For this review, use the dimensioned drawing (mm, ordinates from the lowest corner) and the shaded views. A direction names the side the tool comes from. Round coordinates to 2 decimals unless told otherwise and drop trailing zeros. Loops run counter-clockwise (first coordinate to the right, second up) from the corner with the lowest first, then second, coordinate; pieces in that order, holes last. Notation, with made-up numbers: (10, 45.5) - (34, 45.5) arc R29 ccw to (34, 70.5) - close; hole circle Ø10 at (80.5, 73.25). An arc over 180 degrees is marked (long way). Answer as CSV lines item,"result". Start each with the question number.
(1) For the marked faces 4, 5 and 6, list the 3-axis set-ups (+Z, -Z, +X, -X, +Y, -Y) from which the entire face can be reached by the end or side of a thin tool; tool diameter is ignored.
(2) For P1, Ø2, axis at y = 47.5, z = 2, coming from the +X side; P2, Ø1, axis at y = 53.5, z = 2, coming from the -X side, all flat-tipped, find the tip position at first contact; note any pin that passes through.
(3) Consider section B-B (z = 2.8). Count the separate pieces of the cut face and the enclosed holes in it, and give its area (3 significant figures).
(4) Wall thickness on L1, parallel to Y at x = 20, z = 0.95; L2, parallel to X at y = 68.5, z = 3.85; L3, parallel to Y at x = 35, z = 1.95: over which ranges is each line inside the solid? List them lowest first.
(5) Consider section D-D (y = 75). Give the boundary of the cut face in (x, z), and give its area (3 significant figures).
(6) Consider section A-A (y = 7.5). Give the boundary of the cut face in (x, z), and give its area (3 significant figures).
(7) Consider section C-C (x = 4). Give the boundary of the cut face in (y, z), and give its area (3 significant figures).
(8) Mouldability with a two-part tool opening along X and no side actions: class the marked faces 1, 2 and 3 as released by +X, released by -X, zero draft, split by the parting line, or undercut.
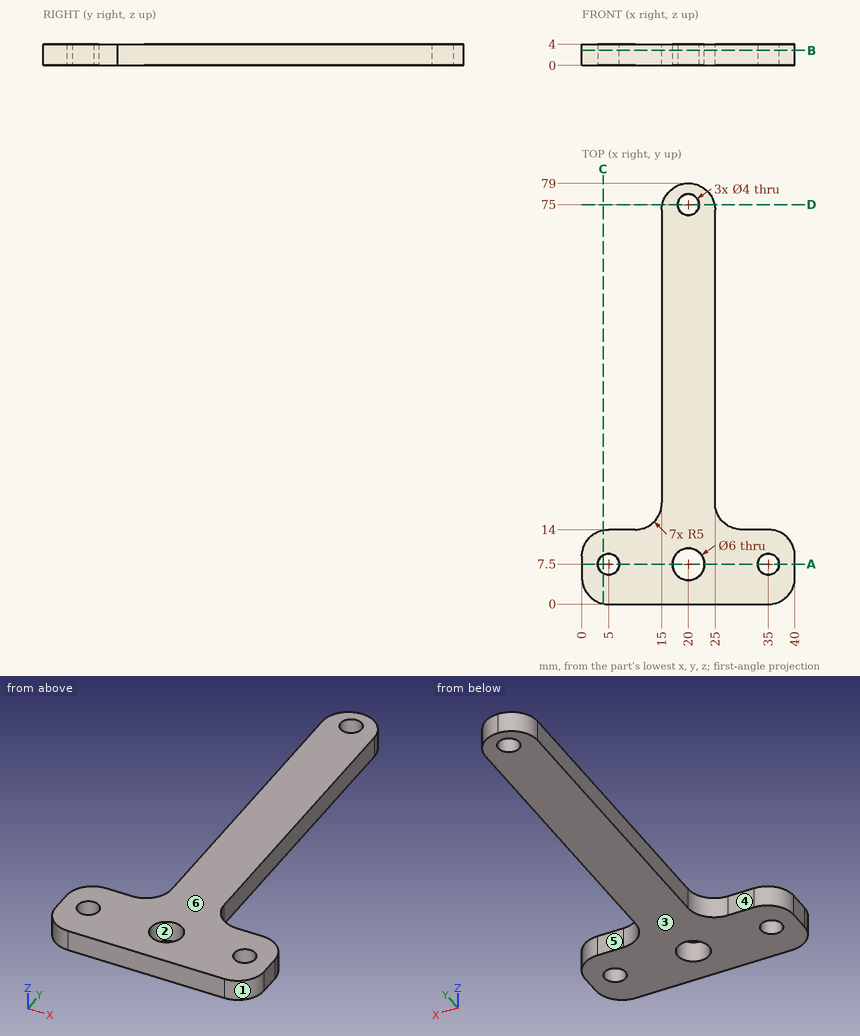
Determined:
1,face 4,"+Z, -Z, -X, +Y"
1,face 5,"+Z, -Z, +X, +Y"
1,face 6,"+Z, +X, -X, +Y, -Y"
2,P1,"stops at x = 25"
2,P2,"stops at x = 15"
3,separate pieces,"1"
3,enclosed holes,"4"
3,area,"1,120 mm^2"
4,L1,"y = 0 to 4.5, 10.5 to 73, 77 to 79"
4,L2,"x = 15 to 25"
4,L3,"y = 0 to 5.5, 9.5 to 14"
5,outline,"(15.1, 0) - (18, 0) - (18, 4) - (15.1, 4) - close; (22, 0) - (24.9, 0) - (24.9, 4) - (22, 4) - close"
5,area,"23.2 mm^2"
6,outline,"(0, 0) - (3, 0) - (3, 4) - (0, 4) - close; (7, 0) - (17, 0) - (17, 4) - (7, 4) - close; (23, 0) - (33, 0) - (33, 4) - (23, 4) - close; (37, 0) - (40, 0) - (40, 4) - (37, 4) - close"
6,area,"104 mm^2"
7,outline,"(0.1, 0) - (5.77, 0) - (5.77, 4) - (0.1, 4) - close; (9.23, 0) - (13.9, 0) - (13.9, 4) - (9.23, 4) - close"
7,area,"41.3 mm^2"
8,face 1,"released by +X"
8,face 2,"undercut"
8,face 3,"zero draft"
